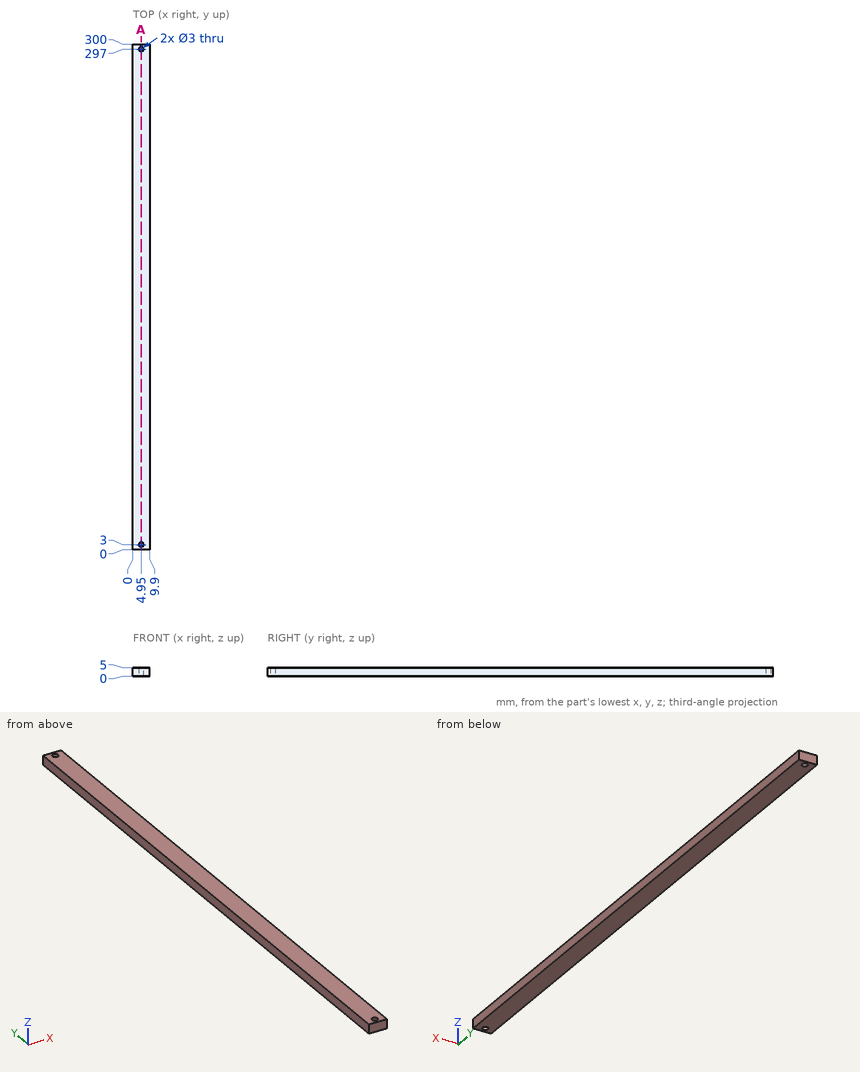
Print and shaded views of the part. All mm, measured from the part's lowest x, y and z. Coordinates: 2 decimals unless noted, no trailing zeros. Loops run counter-clockwise (first coordinate to the right, second up) from the corner with the lowest first, then second, coordinate; pieces in that order, holes last. Notation, with made-up numbers: M -30,-14.75 L 4,-14.75 A19 cw 4,-9.75 Z; hole C -15.75,78 d3. An arc over 180 degrees is marked long. Use a Markdown table: item, result. Add a question column.
Q1. Probe L1, parallel to Y at x = 4.95, z = 3.9; L2, parallel to Y at x = 4, z = 2.2; L3, parallel to X at y = 297, z = 3.95. List the from-to ranges inside material, lowest first.
Q2. Cut at A-A (x = 4.95). Write the cut outline in (y, z).
Q3. Pin check, flat tip, straight feed: P1, Ø1.8, axis at x = 4.95, y = 3, coming from the +Z side. Stop position of the tip, or through.
Worked out:
| question | item | result |
|---|---|---|
| 1 | L1 | y = 0 to 1.5, 4.5 to 295.5, 298.5 to 300 |
| 1 | L2 | y = 0 to 1.84, 4.16 to 295.84, 298.16 to 300 |
| 1 | L3 | x = 0 to 3.45, 6.45 to 9.9 |
| 2 | outline | M 0,0 L 1.5,0 L 1.5,5 L 0,5 Z; M 4.5,0 L 295.5,0 L 295.5,5 L 4.5,5 Z; M 298.5,0 L 300,0 L 300,5 L 298.5,5 Z |
| 3 | P1 | passes through |
